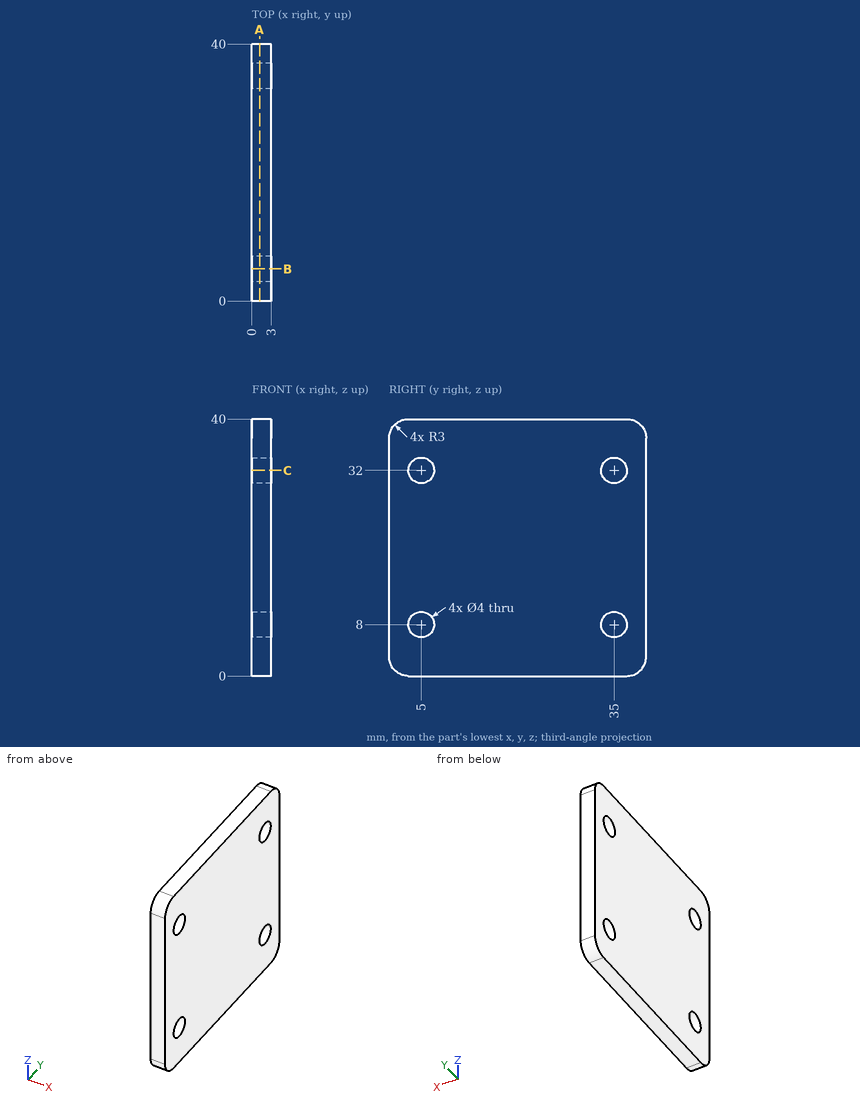
Geometry check sheet. Reference: drawing and pictorial views, mm from the part's lowest x, y, z. Coordinates: 2 decimals unless noted, no trailing zeros. Order: outer loops, then holes, each group sorted by start corner. A loop starts at its lowest first (then second) coordinate and runs counter-clockwise, first axis right, second up. Notation, with made-up numbers: (-38.5, 34.25) -> (-33.5, 34.25) arc R23 ccw to (-33.5, 57.25) -> close; hole circle Ø8 at (51, 29.5). An arc over 180 degrees is marked (long way). Put each result on its own line as item: value. Start each with the question number.
1) Cross-section at C-C (z = 32). Enter the section's corners in (x, y).
2) Material ranges on L1, parallel to Z at x = 2.4, y = 35; L2, parallel to Y at x = 1.45, z = 8; L3, parallel to Y at x = 1.4, z = 31, recorded low to high.
3) Cross-section at A-A (x = 1.2). Enter the section's corners in (y, z), plus the area to 3 significant figures.
4) Cross-section at B-B (y = 5). Enter the section's corners in (x, z), plus the area to 3 significant figures.
Geometry check:
1. outline: (0, 0) -> (3, 0) -> (3, 3) -> (0, 3) -> close; (0, 7) -> (3, 7) -> (3, 33) -> (0, 33) -> close; (0, 37) -> (3, 37) -> (3, 40) -> (0, 40) -> close
2. L1: z = 0 to 6, 10 to 30, 34 to 40
2. L2: y = 0 to 3, 7 to 33, 37 to 40
2. L3: y = 0 to 3.27, 6.73 to 33.27, 36.73 to 40
3. outline: (0, 3) arc R3 ccw to (3, 0) -> (37, 0) arc R3 ccw to (40, 3) -> (40, 37) arc R3 ccw to (37, 40) -> (3, 40) arc R3 ccw to (0, 37) -> close; hole circle Ø4 at (5, 8); hole circle Ø4 at (5, 32); hole circle Ø4 at (35, 8); hole circle Ø4 at (35, 32)
3. area: 1,540 mm^2
4. outline: (0, 0) -> (3, 0) -> (3, 6) -> (0, 6) -> close; (0, 10) -> (3, 10) -> (3, 30) -> (0, 30) -> close; (0, 34) -> (3, 34) -> (3, 40) -> (0, 40) -> close
4. area: 96.0 mm^2
